```python
from build123d import *

# Parameters (mm, degrees)
SKETCH1_W           = 23.83
SKETCH1_H           = 1
BOSS_EXTRUDE1_DEPTH = 16.5
SKETCH2_R           = 1.325
BOSS_EXTRUDE2_DEPTH = 11.75
BOSS_EXTRUDE4_DEPTH = 8
SKETCH5_W           = 21.811051378
SKETCH5_H           = 2.5
BOSS_EXTRUDE5_DEPTH = 45
SKETCH6_R           = 4.25
SKETCH6_R_2         = 1.05
CUT_EXTRUDE1_DEPTH  = 79.646360374
FILLET1_R           = 7
FILLET2_R           = 7
FILLET3_R           = 7
BOSS_EXTRUDE6_START = 41
BOSS_EXTRUDE6_DEPTH = 41


with BuildPart() as part:
    # Sketch1 → Boss-Extrude1 (new body)
    with BuildSketch(Plane(origin=(0, 0, 0), x_dir=(1, 0, 0), z_dir=(0, 1, 0))):
        Rectangle(SKETCH1_W, SKETCH1_H)
    extrude(amount=BOSS_EXTRUDE1_DEPTH)

    # Sketch2 → Boss-Extrude2 (add, symmetric)
    with BuildSketch(Plane(origin=(0, 8.25, 0), x_dir=(1, 0, 0), z_dir=(0, 1, 0))):
        with Locations(Location((-11.915, 0, 0), (0, 0, 270))):
            Circle(SKETCH2_R)
        with Locations(Location((11.915, 0, 0), (0, 0, 270))):
            Circle(SKETCH2_R)
    extrude(amount=BOSS_EXTRUDE2_DEPTH, both=True)

    # Sketch4 → Boss-Extrude4 (add, symmetric)
    with BuildSketch(Plane(origin=(0, 0, 0), x_dir=(0, 0, -1), z_dir=(1, 0, 0))):
        Polygon((-0.5, 12.538583985), (-0.5, 16.5), (-12.5, 31.25), (-35.5, 31.25), (-35.5, 28.75), (-13.688948622, 28.75), align=None)
        Polygon((-0.5, 0), (-0.5, 3.961416015), (-13.688948622, -12.25), (-35.5, -12.25), (-35.5, -14.75), (-12.5, -14.75), align=None)
    extrude(amount=BOSS_EXTRUDE4_DEPTH, both=True)

    # Sketch5 → Boss-Extrude5 (add)
    with BuildSketch(Plane.ZY.offset(8)):
        with Locations((24.594474311, 30)):
            Rectangle(SKETCH5_W, SKETCH5_H)
        with Locations((24.594474311, -13.5)):
            Rectangle(SKETCH5_W, SKETCH5_H)
    extrude(amount=BOSS_EXTRUDE5_DEPTH)

    # Sketch6 → Cut-Extrude1 (cut, through all)
    with BuildSketch(Plane(origin=(0, 31.25, 0), x_dir=(1, 0, 0), z_dir=(0, 1, 0))):
        with Locations(Location((-42.094474311, -24.594474311, 0), (0, 0, 270))):
            Circle(SKETCH6_R)
        with Locations(Location((-49.094474311, -24.594474311, 0), (0, 0, 270))):
            Circle(SKETCH6_R_2)
        with Locations(Location((-42.094474311, -17.594474311, 0), (0, 0, 270))):
            Circle(SKETCH6_R_2)
        with Locations(Location((-35.094474311, -24.594474311, 0), (0, 0, 270))):
            Circle(SKETCH6_R_2)
        with Locations(Location((-42.094474311, -31.594474311, 0), (0, 0, 270))):
            Circle(SKETCH6_R_2)
        with BuildLine():
            ThreePointArc((-53, -24.594474311), (-49.805845478, -16.883103144), (-42.094474311, -13.688948622))
            Line((-42.094474311, -13.688948622), (-53, -13.688948622))
            Line((-53, -13.688948622), (-53, -24.594474311))
        make_face()
        with BuildLine():
            ThreePointArc((-42.094474311, -35.5), (-49.805845478, -32.305845478), (-53, -24.594474311))
            Line((-53, -24.594474311), (-53, -35.5))
            Line((-53, -35.5), (-42.094474311, -35.5))
        make_face()
    extrude(amount=-CUT_EXTRUDE1_DEPTH, mode=Mode.SUBTRACT)

    # Fillet1
    # the kernel refuses this fillet: 7 mm, written as the material it adds along each edge
    with BuildSketch(Plane(origin=(-8, -14.75, 13.688948622), x_dir=(-1, 0, 0), z_dir=(0, 1, 0))) as fillet1_piece_1_section:
        with BuildLine():
            CenterArc((FILLET1_R, -FILLET1_R), FILLET1_R, 90, 90)
            Line((0, -FILLET1_R), (0, 0))
            Line((0, 0), (FILLET1_R, 0))
        make_face()
    fillet1_piece_1 = extrude(amount=2.5, mode=Mode.PRIVATE)
    fillet1_piece_1 = split(fillet1_piece_1, bisect_by=Plane(origin=(-10.031790315, -14.125351158, 11.991811112), z_dir=(0, 0.6310874674162202, 0.7757116786991036)), keep=Keep.TOP, mode=Mode.PRIVATE)
    fillet1_piece_1 = split(fillet1_piece_1, bisect_by=Plane(origin=(-10.031790315, -12.54763249, 13.931090308), z_dir=(0, -0.6310874674162201, -0.7757116786991036)), keep=Keep.TOP, mode=Mode.PRIVATE)
    add(fillet1_piece_1)
    with BuildSketch(Plane(origin=(-8, -14.75, 13.688948622), x_dir=(-1, 0, 0), z_dir=(0, 1, 0))) as fillet1_piece_2_section:
        with BuildLine():
            CenterArc((FILLET1_R, -FILLET1_R), FILLET1_R, 90, 90)
            Line((0, -FILLET1_R), (0, 0))
            Line((0, 0), (FILLET1_R, 0))
        make_face()
    fillet1_piece_2 = extrude(amount=20, mode=Mode.PRIVATE)
    fillet1_piece_2 = split(fillet1_piece_2, bisect_by=Plane(origin=(-8.829123945, -11.325395044, 9.713880714), z_dir=(0, 0.6310874674162202, 0.7757116786991036)), keep=Keep.TOP, mode=Mode.PRIVATE)
    fillet1_piece_2 = split(fillet1_piece_2, bisect_by=Plane(origin=(-8.829123945, -12.25, 10.954048459), z_dir=(0, 1, 0)), keep=Keep.TOP, mode=Mode.PRIVATE)
    fillet1_piece_2 = split(fillet1_piece_2, bisect_by=Plane(origin=(-8.829123945, -9.747676376, 11.653159911), z_dir=(0, -0.6310874674162201, -0.7757116786991036)), keep=Keep.TOP, mode=Mode.PRIVATE)
    add(fillet1_piece_2)
    with BuildSketch(Plane(origin=(-8, 31.25, 13.688948622), x_dir=(0, 0, -1), z_dir=(0, -1, 0))) as fillet1_piece_3_section:
        with BuildLine():
            CenterArc((FILLET1_R, -FILLET1_R), FILLET1_R, 90, 90)
            Line((0, -FILLET1_R), (0, 0))
            Line((0, 0), (FILLET1_R, 0))
        make_face()
    fillet1_piece_3 = extrude(amount=2.5, mode=Mode.PRIVATE)
    fillet1_piece_3 = split(fillet1_piece_3, bisect_by=Plane(origin=(-10.031790315, 29.047632489, 13.931090308), z_dir=(0, 0.6310874674162203, -0.7757116786991034)), keep=Keep.TOP, mode=Mode.PRIVATE)
    fillet1_piece_3 = split(fillet1_piece_3, bisect_by=Plane(origin=(-10.031790315, 30.625351158, 11.991811112), z_dir=(0, -0.6310874674162202, 0.7757116786991036)), keep=Keep.TOP, mode=Mode.PRIVATE)
    add(fillet1_piece_3)
    with BuildSketch(Plane(origin=(-8, 31.25, 13.688948622), x_dir=(0, 0, -1), z_dir=(0, -1, 0))) as fillet1_piece_4_section:
        with BuildLine():
            CenterArc((FILLET1_R, -FILLET1_R), FILLET1_R, 90, 90)
            Line((0, -FILLET1_R), (0, 0))
            Line((0, 0), (FILLET1_R, 0))
        make_face()
    fillet1_piece_4 = extrude(amount=20, mode=Mode.PRIVATE)
    fillet1_piece_4 = split(fillet1_piece_4, bisect_by=Plane(origin=(-8.829123957, 26.247676381, 11.653159915), z_dir=(0, 0.6310874674162203, -0.7757116786991034)), keep=Keep.TOP, mode=Mode.PRIVATE)
    fillet1_piece_4 = split(fillet1_piece_4, bisect_by=Plane(origin=(-8.829123957, 27.82539505, 9.713880718), z_dir=(0, -0.6310874674162202, 0.7757116786991036)), keep=Keep.TOP, mode=Mode.PRIVATE)
    fillet1_piece_4 = split(fillet1_piece_4, bisect_by=Plane(origin=(-8.829123957, 28.75, 10.954048463), z_dir=(0, -1, 0)), keep=Keep.TOP, mode=Mode.PRIVATE)
    add(fillet1_piece_4)
    # the kernel refuses this fillet: 7 mm, written as the material it takes off along each edge
    with BuildSketch(Plane(origin=(8, 5.25, 35.5), x_dir=(0, 0, -1), z_dir=(0, -1, 0))) as fillet1_2_piece_1:
        with BuildLine():
            CenterArc((FILLET1_R, -FILLET1_R), FILLET1_R, 90, 90)
            Line((0, -FILLET1_R), (0, 0))
            Line((0, 0), (FILLET1_R, 0))
        make_face()
    extrude(amount=37.5, mode=Mode.SUBTRACT)
    with BuildSketch(Plane(origin=(8, 48.75, 35.5), x_dir=(-1, 0, 0), z_dir=(0, -1, 0))) as fillet1_2_piece_2:
        with BuildLine():
            CenterArc((FILLET1_R, FILLET1_R), FILLET1_R, 180, 90)
            Line((0, FILLET1_R), (0, 0))
            Line((0, 0), (FILLET1_R, 0))
        make_face()
    extrude(amount=37.5, mode=Mode.SUBTRACT)

    # Fillet2
    fillet2_edges = [part.edges().sort_by_distance(p)[0] for p in [
        (0, 12.538583985, 0.5),
        (0, 3.961416015, 0.5),
    ]]
    fillet(fillet2_edges, radius=FILLET2_R)

    # Fillet3
    # the kernel refuses this fillet: 7 mm, written as the material it adds along each edge
    with BuildSketch(Plane(origin=(-8, 16.5, 0.5), x_dir=(0, 0.7757116786988805, 0.6310874674164945), z_dir=(1, 0, 0))) as fillet3_piece_1:
        with BuildLine():
            CenterArc((2.571760467, -7), FILLET3_R, 90, 27.229107119)
            Line((-0.631087467, -0.775711679), (0, 0))
            Line((0, 0), (2.571760467, 0))
        make_face()
    extrude(amount=16)
    with BuildSketch(Plane(origin=(8, 0, 0.5), x_dir=(0, 0, -1), z_dir=(-1, 0, 0))) as fillet3_piece_2:
        with BuildLine():
            CenterArc((3.806975951, 6.412556901), FILLET3_R, 219.130399557, 27.229107119)
            Line((-1.6230058, 1.994944629), (0, 0))
            Line((0, 0), (1, 0))
        make_face()
    extrude(amount=16)

    # Sketch8 → Boss-Extrude6 (add)
    with BuildSketch(Plane(origin=(0, -12.25, 0), x_dir=(1, 0, 0), z_dir=(0, 1, 0)).offset(BOSS_EXTRUDE6_START)):
        with BuildLine():
            ThreePointArc((1, -35.5), (5.949747468, -33.449747468), (8, -28.5))
            Line((8, -28.5), (5, -28.5))
            ThreePointArc((5, -28.5), (3.422054899, -30.922054899), (1, -32.5))
            Line((1, -32.5), (1, -35.5))
        make_face()
    extrude(amount=-BOSS_EXTRUDE6_DEPTH)


solid = part.part
```
Work out the finished part from the listing and answer in its coordinate system (mm). A direction names the side the tool comes from. Give positions to 0.01 mm unless a question says otherwise; leave off trailing zeros. Write each loop counter-clockwise with the first axis right and the second up, starting at its lowest first coordinate (ties: lowest second). Pieces come first, ordered by that corner, then holes. Notation, with made-up numbers: (66, -5) - (103, -5) arc R15 cw to (103, 5) - close; hole circle Ø5 at (-16.75, 6.25). An arc over 180 degrees is marked (long way). Use one line per item in the form item = value.
1. A cutting plane is placed at A-A (z = 19.5). Write down the section's boundary in (x, y), and give its area (3 significant figures).
Filled in:
outline = (-51.74, -14.75) - (8, -14.75) - (8, -12.25) - (-51.74, -12.25) - close; (-51.74, 28.75) - (8, 28.75) - (8, 31.25) - (-51.74, 31.25) - close
area = 299 mm^2
2. For faces 4 (the face through (0.44, -8.462, 7.384)), 5 (the face through (-0.112, 12.426, 0.915)), determine the directions among +Z, -Z, +X, -X, +Y, -Y from which every point of the face is accessible in a straight line to the end or side of a thin tool.
Filled in:
face_4 = -Z, +X, -X, -Y
face_5 = none
3. A cutting plane is placed at C-C (y = 1). Write down the section's boundary in (x, z) (3 decimals), and give its area (3 significant figures).
Filled in:
outline = (-10.688, -0.5) - (10.688, -0.5) arc R1.325 ccw (long way) to (10.688, 0.5) - (8, 0.5) - (8, 2.909) - (-8, 2.909) - (-8, 0.5) - (-10.688, 0.5) arc R1.325 ccw (long way) to start; (1, 32.5) arc R7 cw to (5, 28.5) - (8, 28.5) arc R7 ccw to (1, 35.5) - close
area = 99.0 mm^2
4. A cutting plane is placed at B-B (x = 4). Write down the section's boundary in (y, z).
Filled in:
outline = (-14.75, 12.5) - (-1.99, 2.12) arc R7 cw to (0, -0.5) - (16.5, -0.5) arc R7 cw to (18.49, 2.12) - (31.25, 12.5) - (31.25, 34.82) - (-14.75, 34.82) - close; hole (-12.25, 13.69) - (2.03, 2.07) arc R7 ccw to (6.45, 0.5) - (10.05, 0.5) arc R7 ccw to (14.47, 2.07) - (28.75, 13.69) - (28.75, 30.27) - (-12.25, 30.27) - close
5. Each of these flat-tipped pins is pushed along its axis until it touches: pin 1 Ø5 at (x, z) = (-42.09, 24.59) entering from -Y; pin 2 Ø13 at (x, y) = (-3, 5) entering from -Z; pin 3 Ø10 at (x, y) = (-1, 24.5) entering from -Z; pin 4 Ø3.5 at (y, z) = (0.5, 34.5) entering from -X. Where does it stop, or does it pass through?
Filled in:
pin_1 = through
pin_2 = -0.5
pin_3 = 2.94
pin_4 = 1
6. A cutting plane is placed at D-D (z = 31.5). Write down the section's boundary in (x, y).
Filled in:
outline = (-50.54, -14.75) - (-43.14, -14.75) - (-43.14, -12.25) - (-50.54, -12.25) - close; (-50.54, 28.75) - (-43.14, 28.75) - (-43.14, 31.25) - (-50.54, 31.25) - close; (-41.05, -14.75) - (7.32, -14.75) - (7.32, 31.25) - (-41.05, 31.25) - (-41.05, 28.75) - (2.77, 28.75) - (2.77, -12.25) - (-41.05, -12.25) - close
7. Determine the mould class of faces 1 (the face through (3.451, 8.537, 30.893)), 2 (the face through (-41.21, 30.02, 18.16)), 3 (the face through (-23, -14.75, 24)) for opening direction Y: released by +Y, released by -Y, zero draft, split by the parting line, or undercut.
Filled in:
face_1 = undercut
face_2 = zero draft
face_3 = released by -Y
8. Consider L1, parallel to Y at x = -36.5, z = 28; L2, parallel to X at y = 29, z = 22.5; L3, parallel to Y at x = 5, z = 10. Determine where each line is inside the solid, lowest interval first.
Filled in:
L1 = -14.75 to -12.25, 28.75 to 31.25
L2 = -52.8 to -45.79, -38.4 to 8
L3 = -11.68 to -7.72, 24.22 to 28.18
